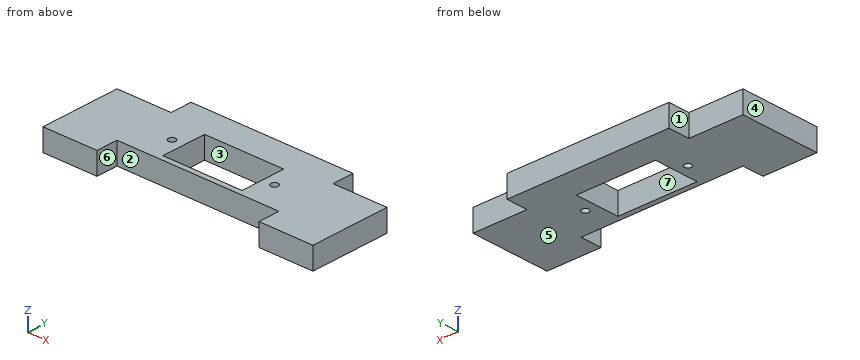
from build123d import *

# Parameters (mm, degrees)
SKETCH1_W                    = 44
SKETCH1_H                    = 25
BOSS_EXTRUDE1_DEPTH          = 12
F_4_0_4_DIAMETER_HOLE1_D     = 4
F_4_0_4_DIAMETER_HOLE1_DEPTH = 25
F_4_0_4_DIAMETER_HOLE1_TIP   = 1.201721238


with BuildPart() as part:
    # Sketch1 → Boss-Extrude1 (new body)
    with BuildSketch(Plane.XY.offset(232.248004761)):
        Polygon((-82.257473883, 114.914823413), (-82.257473883, 82.464823413), (-82.257473883, 70.464823413), (-52.257473883, 70.464823413), (-52.257473883, 82.464823413), (-29.482473883, 82.464823413), (14.967526117, 82.464823413), (37.742526117, 82.464823413), (37.742526117, 70.464823413), (67.742526117, 70.464823413), (67.742526117, 82.464823413), (67.742526117, 114.914823413), (37.742526117, 114.914823413), (37.742526117, 126.914823413), (-52.257473883, 126.914823413), (-52.257473883, 114.914823413), align=None)
        with Locations((-7.482473883, 97.914823413)):
            Rectangle(SKETCH1_W, SKETCH1_H, mode=Mode.SUBTRACT)
    extrude(amount=-BOSS_EXTRUDE1_DEPTH)

    # Ø4.0 (4) Diameter Hole1
    with Locations(Plane(origin=(-7.257473883, 0, 220.248004761), x_dir=(-1, 0, 0), z_dir=(0, 0, -1))):
        with Locations((-28.275, 97.914823413), (28.725, 97.914823413)):
            Hole(F_4_0_4_DIAMETER_HOLE1_D / 2, depth=F_4_0_4_DIAMETER_HOLE1_DEPTH)
            with Locations((0, 0, -(F_4_0_4_DIAMETER_HOLE1_DEPTH + F_4_0_4_DIAMETER_HOLE1_TIP / 2))):  # 118° drill point
                Cone(0, F_4_0_4_DIAMETER_HOLE1_D / 2, F_4_0_4_DIAMETER_HOLE1_TIP, mode=Mode.SUBTRACT)


solid = part.part
Design review of the part built by this model. Coordinates are the model's own, in mm. Face numbers are marked on the shaded views. A direction names the side the tool comes from. Coordinates: 2 decimals unless noted, no trailing zeros. Loops run counter-clockwise (first coordinate to the right, second up) from the corner with the lowest first, then second, coordinate; pieces in that order, holes last.
Item 1: Wall thickness on L1, parallel to X at y = 101.5, z = 227.5; L2, parallel to Y at x = -17.5, z = 226.25; L3, parallel to X at y = 78, z = 224.5: over which ranges is each line inside the solid? List them lowest first.
Completed:
L1: x = -82.26 to -29.48, 14.52 to 67.74
L2: y = 82.46 to 85.41, 110.41 to 126.91
L3: x = -82.26 to -52.26, 37.74 to 67.74
Item 2: Add section D-D (y = 120). Write out the cut boundary in (x, z).
Completed:
outline: (-52.26, 220.25) - (37.74, 220.25) - (37.74, 232.25) - (-52.26, 232.25) - close
Item 3: Add section A-A (y = 77). Write out the cut boundary in (x, z).
Completed:
outline: (-82.26, 220.25) - (-52.26, 220.25) - (-52.26, 232.25) - (-82.26, 232.25) - close; (37.74, 220.25) - (67.74, 220.25) - (67.74, 232.25) - (37.74, 232.25) - close
Item 4: Add section C-C (z = 224.75). Write out the cut boundary in (x, y), and give its area (3 significant figures).
Completed:
outline: (-82.26, 70.46) - (-52.26, 70.46) - (-52.26, 82.46) - (37.74, 82.46) - (37.74, 70.46) - (67.74, 70.46) - (67.74, 114.91) - (37.74, 114.91) - (37.74, 126.91) - (-52.26, 126.91) - (-52.26, 114.91) - (-82.26, 114.91) - close; hole circle Ø4 at (-35.98, 97.91); hole (-29.48, 85.41) - (14.52, 85.41) - (14.52, 110.41) - (-29.48, 110.41) - close; hole circle Ø4 at (21.02, 97.91)
area: 5,540 mm2
Item 5: Clearance check with flat-ended pins moving along their axes: pin 1 (5 mm diameter, centred on x = -45, z = 230, fed in from -Y); pin 2 (6 mm diameter, centred on y = 120, z = 228, fed in from -X); pin 3 (6 mm diameter, centred on y = 120, z = 224.5, fed in from +X). State where each tip first meets the part, or that it passes through.
Completed:
pin 1: stops at y = 82.46
pin 2: stops at x = -52.26
pin 3: stops at x = 37.74
Item 6: Draft analysis for pull direction X (two halves, no side actions). For the marked faces 4, 5, 6 and 7, state which applies: pulls with the +X half, pulls with the -X half, needs draft (parallel to the pull), parting line crosses it, or undercut.
Completed:
face 4: pulls with the -X half
face 5: needs draft
face 6: undercut
face 7: undercut
Item 7: Add section B-B (x = -25). Write out the cut boundary in (y, z), and give its area (3 significant figures).
Completed:
outline: (82.46, 220.25) - (85.41, 220.25) - (85.41, 232.25) - (82.46, 232.25) - close; (110.41, 220.25) - (126.91, 220.25) - (126.91, 232.25) - (110.41, 232.25) - close
area: 233 mm2
Item 8: For the marked faces 1, 2 and 3, list the 3-axis set-ups (+Z, -Z, +X, -X, +Y, -Y) from which the entire face can be reached by the end or side of a thin tool; tool diameter is ignored.
Completed:
face 1: +Z, -Z, -X, +Y
face 2: +Z, -Z, -Y
face 3: +Z, -Z
